Design review of the part built by this model. Coordinates are the model's own, in mm. Face numbers are marked on the shaded views. A direction names the side the tool comes from. Coordinates: 2 decimals unless noted, no trailing zeros. Order: outer loops, then holes, each group sorted by start corner. A loop starts at its lowest first (then second) coordinate and runs counter-clockwise, first axis right, second up. Notation, with made-up numbers: M 78.5,29.5 L 122.5,29.5 A13 ccw 122.5,50.5 Z; hole C 74.5,12.25 d6. An arc over 180 degrees is marked long. Answer as a JSON object with one key per item and string values.
from build123d import *

# Parameters (mm, degrees)
SKETCH1_R           = 37.5
SKETCH1_R_2         = 3
BOSS_EXTRUDE1_DEPTH = 6
FILLET1_R           = 2


with BuildPart() as part:
    # Sketch1 → Boss-Extrude1 (new body)
    with BuildSketch(Plane(origin=(0, 0, 0), x_dir=(0, 0, -1), z_dir=(1, 0, 0))):
        Circle(SKETCH1_R)
        with BuildLine():
            ThreePointArc((-2, 7.745966692), (-6.92820323, 4), (-7.708203932, -2.140932539))
            Line((-7.708203932, -2.140932539), (-29.0924812, -14.487150776))
            ThreePointArc((-29.0924812, -14.487150776), (-28.145825623, 16.25), (-2, 32.438403167))
            Line((-2, 32.438403167), (-2, 7.745966692))
        make_face(mode=Mode.SUBTRACT)
        Circle(SKETCH1_R_2, mode=Mode.SUBTRACT)
        with BuildLine():
            ThreePointArc((-5.708203932, -5.605034154), (0, -8), (5.708203933, -5.605034154))
            Line((5.708203933, -5.605034154), (27.0924812, -17.951252391))
            ThreePointArc((27.0924812, -17.951252391), (0, -32.5), (-27.0924812, -17.951252391))
            Line((-27.0924812, -17.951252391), (-5.708203932, -5.605034154))
        make_face(mode=Mode.SUBTRACT)
        with BuildLine():
            ThreePointArc((7.708203933, -2.140932539), (6.92820323, 4), (2, 7.745966692))
            Line((2, 7.745966692), (2, 32.438403167))
            ThreePointArc((2, 32.438403167), (28.145825623, 16.25), (29.0924812, -14.487150776))
            Line((29.0924812, -14.487150776), (7.708203933, -2.140932539))
        make_face(mode=Mode.SUBTRACT)
    extrude(amount=BOSS_EXTRUDE1_DEPTH)

    # Fillet1
    fillet1_edges = [part.edges().sort_by_distance(p)[0] for p in [
        (3, 32.438403167, 2),
        (3, -14.487150776, 29.0924812),
        (3, -2.140932539, 7.708203932),
        (3, 7.745966692, 2),
        (3, -17.951252391, 27.0924812),
        (3, -17.951252391, -27.0924812),
        (3, -5.605034154, -5.708203933),
        (3, -5.605034154, 5.708203932),
        (3, -14.487150776, -29.0924812),
        (3, 32.438403167, -2),
        (3, 7.745966692, -2),
        (3, -2.140932539, -7.708203933),
    ]]
    fillet(fillet1_edges, radius=FILLET1_R)


solid = part.part
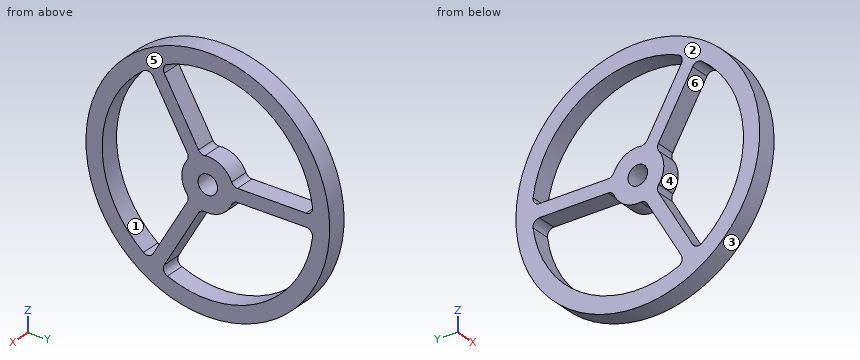
1) Add section D-D (z = 0). State the section outline as (x, y) points, and give its area (3 significant figures).
Taken from the geometry:
{"outline": "M 0,-37.5 L 6,-37.5 L 6,-32.5 L 0,-32.5 Z; M 0,-8 L 6,-8 L 6,-3 L 0,-3 Z; M 0,3 L 6,3 L 6,37.5 L 0,37.5 Z", "area": "267 mm2"}
2) Add section A-A (y = 0). State the section outline as (x, z) points, and give its area (3 significant figures).
Taken from the geometry:
{"outline": "M 0,-37.5 L 6,-37.5 L 6,-32.5 L 0,-32.5 Z; M 0,-8 L 6,-8 L 6,-3 L 0,-3 Z; M 0,3 L 6,3 L 6,8 L 0,8 Z; M 0,32.5 L 6,32.5 L 6,37.5 L 0,37.5 Z", "area": "120 mm2"}
3) To check wall thickness, follow L1, parallel to Y at x = 1.4, z = 0; L2, parallel to Y at x = 4.8, z = 4; L3, parallel to Z at x = 4.45, y = -4. State the ranges of each line that lie inside material, in increasing order.
Taken from the geometry:
{"L1": "y = -37.5 to -32.5, -8 to -3, 3 to 37.5", "L2": "y = -37.29 to -32.25, -6.93 to 6.93, 32.24 to 37.29", "L3": "z = -37.29 to -32.25, -10.93 to 10.93, 32.25 to 37.29"}
4) Insertion check: pin 1 Ø1 at (x, z) = (2, -21) entering from -Y; pin 2 Ø3 at (x, y) = (2, 18.5) entering from +Z; pin 3 Ø3 at (x, y) = (3.5, 24) entering from -Z. Each pin has a flat end and moves straight along its axis. Give the tip position at first contact, or say it passes through.
Taken from the geometry:
{"pin 1": "stops at y = -31.4", "pin 2": "stops at z = 33.43", "pin 3": "stops at z = -30"}
5) Mouldability with a two-part tool opening along Z and no side actions: class the marked faces 1, 2, 3 and 4 as released by +Z, released by -Z, zero draft, split by the parting line, or undercut.
Taken from the geometry:
{"face 1": "undercut", "face 2": "zero draft", "face 3": "split by the parting line", "face 4": "undercut"}
6) Add section B-B (z = -29). State the section outline as (x, y) points, and give its area (3 significant figures).
Taken from the geometry:
{"outline": "M 0,-23.77 L 6,-23.77 L 6,-13.48 L 0,-13.48 Z; M 0,14.67 L 6,14.67 L 6,23.77 L 0,23.77 Z", "area": "116 mm2"}
7) Add section C-C (x = 2.2). State the section outline as (y, z) points, and give its area (3 significant figures).
Taken from the geometry:
{"outline": "C 0,0 d75; hole M -19.8,-25.77 A2 ccw -16.85,-25.19 L -6.31,-6.94 A2 ccw -6.44,-4.75 A8 cw -6.44,4.75 A2 ccw -6.31,6.94 L -16.85,25.19 A2 ccw -19.8,25.77 A32.5 ccw Z; hole M -13.39,-27.19 A2 ccw -12.42,-30.03 A32.5 ccw 32.22,-4.26 A2 ccw 30.24,-2 L 9.17,-2 A2 ccw 7.33,-3.2 A8 cw -0.89,-7.95 A2 ccw -2.85,-8.94 Z; hole M -13.39,27.19 L -2.85,8.94 A2 ccw -0.89,7.95 A8 cw 7.33,3.2 A2 ccw 9.17,2 L 30.24,2 A2 ccw 32.22,4.26 A32.5 ccw -12.42,30.03 A2 ccw Z; hole C 0,0 d6", "area": "1,580 mm2"}
8) Tool access review of the marked faces 5 and 6: name each direction out of +Z, -Z, +X, -X, +Y, -Y from which nothing blocks a thin tool from reaching the whole face with its end or side.
Taken from the geometry:
{"face 5": "+Z, -Z, +X, +Y, -Y", "face 6": "+X, -X"}
